The model under review builds one solid part; all positions refer to its coordinate system, in mm. Round coordinates to 2 decimals unless told otherwise and drop trailing zeros. Loops run counter-clockwise (first coordinate to the right, second up) from the corner with the lowest first, then second, coordinate; pieces in that order, holes last. Notation, with made-up numbers: (88.25, 15) -> (122.25, 15) arc R20 ccw to (122.25, 22) -> close; hole circle Ø9 at (48.25, 50). An arc over 180 degrees is marked (long way). Write each question's results on one line, items separated by ' | '. Start each with the question number.
Item 1: We need section A-A (y = -1.7). Give the boundary of the cut face in (x, z).
Item 2: Mouldability with a two-part tool opening along Z and no side actions: class faces 1 (the flat face through (-2, 2, 4)), 2 (the flat face through (-4, -2.5, -4)), 3 (the cylindrical face through (-5.158, -0.031, -3.955)) as pulls with the +Z half, pulls with the -Z half, needs draft (parallel to the pull), parting line crosses it, or undercut.
Item 3: For L1, parallel to Z at x = 0, y = 2.1; L2, parallel to Z at x = 0, y = -1.3; L3, parallel to X at y = -2.25, z = 4.5, list the stretches that pass through material, from the lowest coordinate up. Write a range as from..to.
from build123d import *

# Parameters (mm, degrees)
F1_R     = 6.5
F1_R_2   = 5.2
F2_DEPTH = 2.5
F1_R_3   = 4.3
F1_R_4   = 3
F3_DEPTH = 2
F4_SIZE  = 0.3


with BuildPart() as f2:
    # F1 (on Front) → F2 (new body, symmetric)
    with BuildSketch(Plane.XZ):
        Circle(F1_R)
        Circle(F1_R_2, mode=Mode.SUBTRACT)
    extrude(amount=F2_DEPTH, both=True)



with BuildPart() as f2b:
    # F1 (on Front) → F2, piece 2 (new body, symmetric)
    with BuildSketch(Plane.XZ):
        Circle(F1_R_3)
        Circle(F1_R_4, mode=Mode.SUBTRACT)
    extrude(amount=F2_DEPTH, both=True)


with BuildPart() as f2_1:
    add(f2.part)

    add(f2b.part)  # F3 merges F2b
    # F1 (on Front) → F3 (join, symmetric)
    with BuildSketch(Plane.XZ):
        Circle(F1_R_2)
        Circle(F1_R_3, mode=Mode.SUBTRACT)
    extrude(amount=F3_DEPTH, both=True)

    # F4
    f4_edges = [f2_1.edges().sort_by_distance(p)[0] for p in [
        (-6.5, -2.5, 0),
        (-5.2, -2.5, 0),
        (-4.3, -2.5, 0),
        (-3, -2.5, 0),
        (-6.5, 2.5, 0),
        (-5.2, 2.5, 0),
        (-4.3, 2.5, 0),
        (-3, 2.5, 0),
    ]]
    chamfer(f4_edges, length=F4_SIZE)


solid = f2_1.part
Here are the results:
1) outline: circle Ø13 at (0, 0); hole circle Ø6 at (0, 0)
2) face 1: undercut | face 2: needs draft | face 3: parting line crosses it
3) L1: z = -6.5..-5.2, -4.3..-3, 3..4.3, 5.2..6.5 | L2: z = -6.5..-3, 3..6.5 | L3: x = -4.62..-2.7, 2.7..4.62
